The model under review builds one solid part; all positions refer to its coordinate system, in mm. A direction names the side the tool comes from. Round coordinates to 2 decimals unless told otherwise and drop trailing zeros. Order: outer loops, then holes, each group sorted by start corner. A loop starts at its lowest first (then second) coordinate and runs counter-clockwise, first axis right, second up. Notation, with made-up numbers: M 81,80 L 135,80 A8 ccw 135,85 Z; hole C 79,43.25 d7. An arc over 180 degrees is marked long. Answer as a JSON object with one key per item and string values. Group by question number.
1) Consider section C-C, the plane z = 12.25. Write out the cut boundary in (x, y), then the cut area to 3 significant figures.
2) Consider section D-D, the plane y = 4. Write out the cut boundary in (x, z).
3) The part is to be moulded in two halves that separate along Y. For faces 1 (the flat face through (35, 41, 15)), 2 (the cylindrical face through (-5.5, -43.07, 2.46)), 3 (the cylindrical face through (48.775, 39.536, 2.535)), say which applies: +Y half, -Y half, draft (parallel to the pull), parting line (faces both ways), or undercut.
4) For faces 4 (the flat face through (33, 44.5, 2)), 5 (the cylindrical face through (0.57, -36.9, 2.46)), list the 3-axis set-ups (+Z, -Z, +X, -X, +Y, -Y) from which the entire face can be reached by the end or side of a thin tool; tool diameter is ignored.
5) Consider section B-B, the plane x = 9. Write out the cut boundary in (y, z).
6) Consider section A-A, the plane x = 56.3. Write out the cut boundary in (y, z), then the cut area to 3 significant figures.
7) To check wall thickness, follow line 1 (Y direction, x = 49.1, z = 4.05); line 2 (Y direction, x = -2.5, z = 3.75); line 3 (Y direction, x = -3.5, z = 2.8). State the ranges of each line that lie inside material, in increasing order.
8) Insertion check: pin 1 Ø3.5 at (x, y) = (56.3, -40.8) entering from +Z; pin 2 Ø2.5 at (x, y) = (-3.5, -20.8) entering from +Z; pin 3 Ø1.5 at (y, z) = (0, 2) entering from +X; pin 4 Ø1.2 at (x, y) = (-3.5, 41) entering from +Z. Each pin has a flat end and moves straight along its axis. Give the tip position at first contact, or say it passes through.
```python
from build123d import *

# Parameters (mm, degrees)
BOSS_EXTRUDE1_DEPTH = 5
SKETCH2_R           = 3
BOSS_EXTRUDE2_DEPTH = 10
SKETCH3_R           = 1.5
CUT_EXTRUDE1_DEPTH  = 6
SKETCH4_R           = 0.77
CUT_EXTRUDE2_DEPTH  = 3


with BuildPart() as part:
    # Sketch1 → Boss-Extrude1 (new body)
    with BuildSketch(Plane.XY):
        with BuildLine():
            Line((0, 35.5), (0, -35.5))
            ThreePointArc((0, -35.5), (0.585786438, -36.914213562), (2, -37.5))
            Line((2, -37.5), (69, -37.5))
            ThreePointArc((69, -37.5), (70.414213562, -38.085786438), (71, -39.5))
            Line((71, -39.5), (71, -42.5))
            ThreePointArc((71, -42.5), (70.414213562, -43.914213562), (69, -44.5))
            Line((69, -44.5), (-2, -44.5))
            ThreePointArc((-2, -44.5), (-5.535533906, -43.035533906), (-7, -39.5))
            Line((-7, -39.5), (-7, 39.5))
            ThreePointArc((-7, 39.5), (-5.535533906, 43.035533906), (-2, 44.5))
            Line((-2, 44.5), (69, 44.5))
            ThreePointArc((69, 44.5), (70.414213562, 43.914213562), (71, 42.5))
            Line((71, 42.5), (71, 39.5))
            ThreePointArc((71, 39.5), (70.414213562, 38.085786438), (69, 37.5))
            Line((69, 37.5), (2, 37.5))
            ThreePointArc((2, 37.5), (0.585786438, 36.914213562), (0, 35.5))
        make_face()
    extrude(amount=BOSS_EXTRUDE1_DEPTH)

    # Sketch2 → Boss-Extrude2 (add)
    with BuildSketch(Plane.XY.offset(5)):
        with Locations((35.1, 41)):
            Circle(SKETCH2_R)
    extrude(amount=BOSS_EXTRUDE2_DEPTH)

    # Sketch3 → Cut-Extrude1 (cut, through all)
    with BuildSketch(Plane.XY.offset(5)):
        with Locations((49.1, 41)):
            Circle(SKETCH3_R)
        with Locations((21.1, 41)):
            Circle(SKETCH3_R)
        with Locations((-3.5, 19)):
            Circle(SKETCH3_R)
        with Locations((-3.5, -20.8)):
            Circle(SKETCH3_R)
        with Locations((27.1, -40.8)):
            Circle(SKETCH3_R)
        with Locations((56.3, -40.8)):
            Circle(SKETCH3_R)
    extrude(amount=-CUT_EXTRUDE1_DEPTH, mode=Mode.SUBTRACT)

    # Sketch4 → Cut-Extrude2 (cut)
    with BuildSketch(Plane.XY.offset(5)):
        with Locations((-3.5, 0)):
            Circle(SKETCH4_R)
        with Locations((-3.5, 41)):
            Circle(SKETCH4_R)
        with Locations((-3.5, -40.8)):
            Circle(SKETCH4_R)
    extrude(amount=-CUT_EXTRUDE2_DEPTH, mode=Mode.SUBTRACT)


solid = part.part
```
Results list:
{
 "1": {"outline": "C 35.1,41 d6", "area": "28.3 mm^2"},
 "2": {"outline": "M -7,0 L 0,0 L 0,5 L -7,5 Z"},
 "3": {"face 1": "draft", "face 2": "-Y half", "face 3": "undercut"},
 "4": {"face 4": "+Z, -Z, +X, -X, +Y", "face 5": "+Z, -Z, +X"},
 "5": {"outline": "M -44.5,0 L -37.5,0 L -37.5,5 L -44.5,5 Z; M 37.5,0 L 44.5,0 L 44.5,5 L 37.5,5 Z"},
 "6": {"outline": "M -44.5,0 L -42.3,0 L -42.3,5 L -44.5,5 Z; M -39.3,0 L -37.5,0 L -37.5,5 L -39.3,5 Z; M 37.5,0 L 44.5,0 L 44.5,5 L 37.5,5 Z", "area": "55.0 mm^2"},
 "7": {"line 1": "-44.5 to -37.5, 37.5 to 39.5, 42.5 to 44.5", "line 2": "-44.47 to -21.92, -19.68 to 17.88, 20.12 to 44.47", "line 3": "-44.27 to -41.57, -40.03 to -22.3, -19.3 to -0.77, 0.77 to 17.5, 20.5 to 40.23, 41.77 to 44.27"},
 "8": {"pin 1": "z = 5", "pin 2": "through", "pin 3": "x = 0", "pin 4": "z = 2"}
}
